The model under review builds one solid part; all positions refer to its coordinate system, in mm. A direction names the side the tool comes from. Give positions to 0.01 mm unless a question says otherwise; leave off trailing zeros. Write each loop counter-clockwise with the first axis right and the second up, starting at its lowest first coordinate (ties: lowest second). Pieces come first, ordered by that corner, then holes.
from build123d import *

# Parameters (mm, degrees)
SALIENTE_EXTRUIR1_DEPTH = 20
CROQUIS4_OUTSIDE_W      = 95.61
CROQUIS4_OUTSIDE_H      = 93.876
CORTAR_EXTRUIR3_DEPTH   = 20


with BuildPart() as part:
    # Croquis1 → Revolución1 (revolve)
    with BuildSketch(Plane(origin=(0, 0, 0), x_dir=(1, 0, 0), z_dir=(0, 1, 0))):
        Polygon((16.7, -87.44), (16.7, 17.5), (20, 17.5), (20, 0), (29, 0), (29, -20), (25, -20), (25, -130), (16.7, -130), align=None)
    revolve(axis=Axis((0, 0, -40.16), (0, 0, 1)))

    # Croquis3 → Saliente-Extruir1 (add)
    with BuildSketch(Plane.XY):
        Polygon((29.866932707, 0), (14.933466354, 25.865522458), (-14.933466354, 25.865522458), (-29.866932707, 0), (-14.933466354, -25.865522458), (14.933466354, -25.865522458), align=None)
    extrude(amount=SALIENTE_EXTRUIR1_DEPTH)

    # Croquis4 outside → Cortar-Extruir3 (cut)
    with BuildSketch(Plane.XY):
        Rectangle(CROQUIS4_OUTSIDE_W, CROQUIS4_OUTSIDE_H)
        Polygon((29.899549638, 0), (14.949774819, 25.893769548), (-14.949774819, 25.893769548), (-29.899549638, 0), (-14.949774819, -25.893769548), (14.949774819, -25.893769548), align=None, mode=Mode.SUBTRACT)
    extrude(amount=CORTAR_EXTRUIR3_DEPTH, mode=Mode.SUBTRACT)


solid = part.part
1) Tool access review of faces 4 (the flat face through (0, 0, 0)), 5 (the flat face through (22.33, -13.11, 9.86)), 6 (the cylindrical face through (15.929, 5.016, 75.77)): name each direction out of +Z, -Z, +X, -X, +Y, -Y from which nothing blocks a thin tool from reaching the whole face with its end or side.
2) Consider section A-A, the plane x = 0. Give the boundary of the cut face in (y, z).
3) To check wall thickness, follow probe 1 along Y at (x, z) = (0, -4); probe 2 along Y at (x, z) = (0, 74); probe 3 along X at (y, z) = (-0.5, 48) (3 decimals). State the ranges of each line that lie inside material, in increasing order.
4) Consider section D-D, the plane y = 22.5. Give the boundary of the cut face in (x, z), then the cut area to 3 significant figures.
5) The part is to be moulded in two halves that separate along X. For faces 1 (the cylindrical face through (23.846, 7.509, 75.77)), 2 (the flat face through (20, 4, 0)), 3 (the flat face through (0, 0, 20)), say which applies: +X half, -X half, draft (parallel to the pull), parting line (faces both ways), or undercut.
6) Consider section B-B, the plane z = -1.5. Give the boundary of the cut face in (x, y), then the cut area to 3 significant figures.
7) Consider section C-C, the plane y = 10.5. Give the boundary of the cut face in (x, z).
8) Insertion check: pin 1 (8 mm diameter, centred on x = -9.5, y = 2.5, fed in from +Z); pin 2 (1.5 mm diameter, centred on y = 3.5, z = 47.5, fed in from -X); pin 3 (16.5 mm diameter, centred on x = -0.5, y = -2.5, fed in from -Z). Each pin has a flat end and moves straight along its axis. Give the tip position at first contact, or say it passes through.
Answer block:
1. face 4: -Z
1. face 5: +Z, -Z, +X, -Y
1. face 6: +Z
2. outline: (-25.89, 0) - (-20, 0) - (-20, -17.5) - (-16.7, -17.5) - (-16.7, 0) - (16.7, 0) - (16.7, -17.5) - (20, -17.5) - (20, 0) - (25.89, 0) - (25.89, 20) - (25, 20) - (25, 130) - (16.7, 130) - (16.7, 20) - (-16.7, 20) - (-16.7, 130) - (-25, 130) - (-25, 20) - (-25.89, 20) - close
3. probe 1: y = -20 to -16.7, 16.7 to 20
3. probe 2: y = -25 to -16.7, 16.7 to 25
3. probe 3: x = -24.995 to -16.693, 16.693 to 24.995
4. outline: (-16.91, 0) - (16.91, 0) - (16.91, 20) - (10.9, 20) - (10.9, 130) - (-10.9, 130) - (-10.9, 20) - (-16.91, 20) - close
4. area: 3,070 mm2
5. face 1: parting line
5. face 2: draft
5. face 3: undercut
6. outline: circle Ø40 at (0, 0); hole circle Ø33.4 at (0, 0)
6. area: 380 mm2
7. outline: (-23.84, 0) - (-17.02, 0) - (-17.02, -17.5) - (-12.99, -17.5) - (-12.99, 0) - (12.99, 0) - (12.99, -17.5) - (17.02, -17.5) - (17.02, 0) - (23.84, 0) - (23.84, 20) - (22.69, 20) - (22.69, 130) - (12.99, 130) - (12.99, 20) - (-12.99, 20) - (-12.99, 130) - (-22.69, 130) - (-22.69, 20) - (-23.84, 20) - close
8. pin 1: stops at z = 20
8. pin 2: stops at x = -24.85
8. pin 3: stops at z = 0
